from build123d import *

# Parameters (mm, degrees)
SKETCH_1_W                   = 50
SKETCH_1_H                   = 30
EXTRUDE_1_DEPTH              = 1
SKETCH_1_3_R                 = 3
EXTRUDE_2_DEPTH              = 5.8
HOLE_WIZARD_M3_1_D           = 3.4
HOLE_WIZARD_M3_1_DEPTH       = 7.5
HOLE_WIZARD_M3_1_CSINK_D     = 6.4
HOLE_WIZARD_M3_1_CSINK_ANGLE = 90
HOLE_WIZARD_M3_1_TIP         = 1.021463052
CHAMFER_1_SIZE               = 1
FILLET_1_R                   = 5


with BuildPart() as part:
    # Sketch 1 → Extrude 1 (new body)
    with BuildSketch(Plane(origin=(0, 0, 0), x_dir=(1, 0, 0), z_dir=(0, 1, 0))):
        Rectangle(SKETCH_1_W, SKETCH_1_H)
    extrude(amount=EXTRUDE_1_DEPTH)

    # Sketch 1_3 → Extrude 2 (add)
    with BuildSketch(Plane(origin=(0, 0, 0), x_dir=(1, 0, 0), z_dir=(0, 1, 0))):
        with Locations(Location((-17.5, 5.75, 0), (0, 0, 270))):
            Circle(SKETCH_1_3_R)
        with Locations(Location((17.5, 5.75, 0), (0, 0, 270))):
            Circle(SKETCH_1_3_R)
        with Locations(Location((0, -5.75, 0), (0, 0, 270))):
            Circle(SKETCH_1_3_R)
    extrude(amount=EXTRUDE_2_DEPTH)

    # Hole Wizard M3 _1
    with Locations(Plane(origin=(0, 0, 0), x_dir=(-1, 0, 0), z_dir=(0, -1, 0))):
        with Locations((-17.5, 5.75), (0, -5.75), (17.5, 5.75)):
            CounterSinkHole(HOLE_WIZARD_M3_1_D / 2, HOLE_WIZARD_M3_1_CSINK_D / 2, depth=HOLE_WIZARD_M3_1_DEPTH, counter_sink_angle=HOLE_WIZARD_M3_1_CSINK_ANGLE)
            with Locations((0, 0, -(HOLE_WIZARD_M3_1_DEPTH + HOLE_WIZARD_M3_1_TIP / 2))):  # 118° drill point
                Cone(0, HOLE_WIZARD_M3_1_D / 2, HOLE_WIZARD_M3_1_TIP, mode=Mode.SUBTRACT)

    # Chamfer 1
    chamfer_1_edges = [part.edges().sort_by_distance(p)[0] for p in [
        (-17.5, 5.8, -8.75),
        (17.5, 5.8, -8.75),
        (0, 5.8, 2.75),
    ]]
    chamfer(chamfer_1_edges, length=CHAMFER_1_SIZE)

    # Fillet 1
    fillet_1_edges = [part.edges().sort_by_distance(p)[0] for p in [
        (-25, 0.5, -15),
        (25, 0.5, -15),
        (25, 0.5, 15),
        (-25, 0.5, 15),
    ]]
    fillet(fillet_1_edges, radius=FILLET_1_R)


solid = part.part
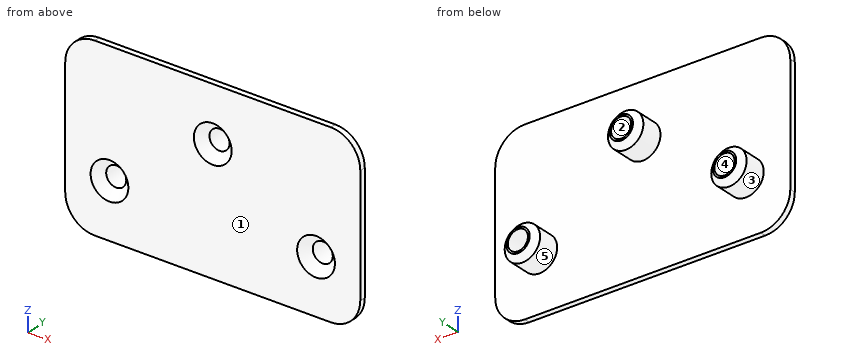
Part model, mm, in its own coordinate system. Face numbers are marked on the shaded views. A direction names the side the tool comes from. Give positions to 0.01 mm unless a question says otherwise; leave off trailing zeros. Write each loop counter-clockwise with the first axis right and the second up, starting at its lowest first coordinate (ties: lowest second). Pieces come first, ordered by that corner, then holes.
1) Cut at A-A on y = 2.9. Write the cut outline in (x, z), then the cut area to 3 significant figures.
Resolved:
outline: circle Ø6 at (-17.5, -5.75); circle Ø6 at (0, 5.75); circle Ø6 at (17.5, -5.75); hole circle Ø3.4 at (-17.5, -5.75); hole circle Ø3.4 at (0, 5.75); hole circle Ø3.4 at (17.5, -5.75)
area: 57.6 mm2
2) Pin check, flat tips, straight feed: pin 1 (2 mm diameter, centred on x = 0, z = 5.75, fed in from -Y); pin 2 (2 mm diameter, centred on x = 12, z = 10.5, fed in from +Y). Stop position of each tip, or through.
Resolved:
pin 1: passes through
pin 2: stops at y = 1
3) Two-plate mould, pull along Z, no slides. Class the marked faces 1, 2 and 3: released by +Z, released by -Z, zero draft, split by the parting line, or undercut.
Resolved:
face 1: zero draft
face 2: undercut
face 3: split by the parting line
4) Probe L1, parallel to X at y = 4.75, z = -5.75; L2, parallel to Z at x = 17.5, y = 2.4; L3, parallel to Y at x = -10, z = 2.75. List the from-to ranges inside material, lowest first.
Resolved:
L1: x = -20.5 to -19.2, -15.8 to -14.5, 14.5 to 15.8, 19.2 to 20.5
L2: z = -8.75 to -7.45, -4.05 to -2.75
L3: y = 0 to 1
5) Cut at C-C on x = 17.5. Write the cut outline in (y, z).
Resolved:
outline: (0, -15) - (1, -15) - (1, -8.75) - (4.8, -8.75) - (5.8, -7.75) - (5.8, -7.45) - (1.5, -7.45) - (0, -8.95) - close; (0, -2.55) - (1.5, -4.05) - (5.8, -4.05) - (5.8, -3.75) - (4.8, -2.75) - (1, -2.75) - (1, 15) - (0, 15) - close
6) Which spindle directions (+Z, -Z, +X, -X, +Y, -Y) get a long thin tool onto all of the face, cutting with end or side? Do the marked faces 4 and 5. Say none if no direction does.
Resolved:
face 4: +Y, -Y
face 5: +Y
7) Cut at B-B on z = -5.75. Write the cut outline in (x, y), then the cut area to 3 significant figures.
Resolved:
outline: (-25, 0) - (-20.7, 0) - (-19.2, 1.5) - (-19.2, 5.8) - (-19.5, 5.8) - (-20.5, 4.8) - (-20.5, 1) - (-25, 1) - close; (-15.8, 1.5) - (-14.3, 0) - (14.3, 0) - (15.8, 1.5) - (15.8, 5.8) - (15.5, 5.8) - (14.5, 4.8) - (14.5, 1) - (-14.5, 1) - (-14.5, 4.8) - (-15.5, 5.8) - (-15.8, 5.8) - close; (19.2, 1.5) - (20.7, 0) - (25, 0) - (25, 1) - (20.5, 1) - (20.5, 4.8) - (19.5, 5.8) - (19.2, 5.8) - close
area: 61.7 mm2
8) Cut at D-D on z = 5.75. Write the cut outline in (x, y), then the cut area to 3 significant figures.
Resolved:
outline: (-25, 0) - (-3.2, 0) - (-1.7, 1.5) - (-1.7, 5.8) - (-2, 5.8) - (-3, 4.8) - (-3, 1) - (-25, 1) - close; (1.7, 1.5) - (3.2, 0) - (25, 0) - (25, 1) - (3, 1) - (3, 4.8) - (2, 5.8) - (1.7, 5.8) - close
area: 55.8 mm2
